```python
from build123d import *

# Parameters (mm, degrees)
ESQUISSE1_W             = 100
ESQUISSE1_H             = 3
BOSS_EXTRU_1_DEPTH      = 338
ESQUISSE2_W             = 12
ESQUISSE2_H             = 6
ESQUISSE2_W_2           = 2
ESQUISSE2_W_3           = 10
ENL_V_MAT_EXTRU_1_DEPTH = 6
ESQUISSE3_W             = 8
ESQUISSE3_H             = 3
BOSS_EXTRU_2_DEPTH      = 6
ESQUISSE4_W             = 42.5
ESQUISSE4_H             = 30
ESQUISSE4_W_2           = 32.5
ENL_V_MAT_EXTRU_2_DEPTH = 10


with BuildPart() as part:
    # Esquisse1 → Boss.-Extru.1 (new body)
    with BuildSketch(Plane.XY):
        with Locations((50, 1.5)):
            Rectangle(ESQUISSE1_W, ESQUISSE1_H)
    extrude(amount=BOSS_EXTRU_1_DEPTH)

    # Esquisse2 → Enlèv. mat.-Extru.1 (cut)
    with BuildSketch(Plane.XZ):
        with Locations((44, 43)):
            Rectangle(ESQUISSE2_W, ESQUISSE2_H)
        with Locations((24, 43)):
            Rectangle(ESQUISSE2_W, ESQUISSE2_H)
        with Locations((64, 43)):
            Rectangle(ESQUISSE2_W, ESQUISSE2_H)
        with Locations((84, 43)):
            Rectangle(ESQUISSE2_W, ESQUISSE2_H)
        with Locations((99, 43)):
            Rectangle(ESQUISSE2_W_2, ESQUISSE2_H)
        with Locations((5, 43)):
            Rectangle(ESQUISSE2_W_3, ESQUISSE2_H)
    extrude(amount=-ENL_V_MAT_EXTRU_1_DEPTH, mode=Mode.SUBTRACT)

    # Esquisse3 → Boss.-Extru.2 (add)
    with BuildSketch(Plane(origin=(0, 0, 0), x_dir=(-1, 0, 0), z_dir=(0, 0, -1))):
        with Locations((-15, 1.5)):
            Rectangle(ESQUISSE3_W, ESQUISSE3_H)
        with Locations((-35, 1.5)):
            Rectangle(ESQUISSE3_W, ESQUISSE3_H)
        with Locations((-55, 1.5)):
            Rectangle(ESQUISSE3_W, ESQUISSE3_H)
        with Locations((-75, 1.5)):
            Rectangle(ESQUISSE3_W, ESQUISSE3_H)
        with Locations((-95, 1.5)):
            Rectangle(ESQUISSE3_W, ESQUISSE3_H)
    boss_extru_2 = extrude(amount=BOSS_EXTRU_2_DEPTH)

    # Symétrie1: Boss.-Extru.2 across plane
    add(boss_extru_2.mirror(Plane(origin=(0, 0, 169), x_dir=(1, 0, 0), z_dir=(0, 0, -1))))

    # Esquisse4 → Enlèv. mat.-Extru.2 (cut)
    with BuildSketch(Plane.XZ):
        with Locations((31.25, 20)):
            Rectangle(ESQUISSE4_W, ESQUISSE4_H)
        with Locations((73.75, 20)):
            Rectangle(ESQUISSE4_W_2, ESQUISSE4_H)
    extrude(amount=-ENL_V_MAT_EXTRU_2_DEPTH, mode=Mode.SUBTRACT)


solid = part.part
```
Geometry: final body of the model. Coordinates: model frame, mm. Give positions to 0.01 mm unless a question says otherwise; leave off trailing zeros. Write each loop counter-clockwise with the first axis right and the second up, starting at its lowest first coordinate (ties: lowest second). Pieces come first, ordered by that corner, then holes.
1. Section query A-A, the plane x = 47. Return loops of the section in (y, z), then the cut area to 3 significant figures.
2. Section query B-B, the plane y = 0.9. Count the separate pieces of the cut face and the enclosed holes in it, then the cut area to 3 significant figures.
3. Pin query (flat end, axial travel): P1, Ø0.9, axis at y = 2, z = -3, coming from the -X side; P2, Ø0.5, axis at x = 99.5, y = 2, coming from the +Z side; P3, Ø1.5, axis at y = 1, z = -2, coming from the +X side. Return the tip coordinate at first contact, or that it passes through.
4. Line query: probe 1 along Z at (x, y) = (43, 0.35); probe 2 along X at (y, z) = (2.9, 23); probe 3 along Z at (x, y) = (9.5, 0.8). Output: solid intervals per line, ascending.
Computed:
1. outline: (0, 0) - (3, 0) - (3, 5) - (0, 5) - close; (0, 35) - (3, 35) - (3, 40) - (0, 40) - close; (0, 46) - (3, 46) - (3, 338) - (0, 338) - close
1. area: 906 mm2
2. separate pieces: 1
2. enclosed holes: 6
2. area: 31,700 mm2
3. P1: stops at x = 11
3. P2: stops at z = 338
3. P3: stops at x = 99
4. probe 1: z = 0 to 5, 35 to 40, 46 to 338
4. probe 2: x = 0 to 10, 52.5 to 57.5, 90 to 100
4. probe 3: z = 0 to 40, 46 to 338
